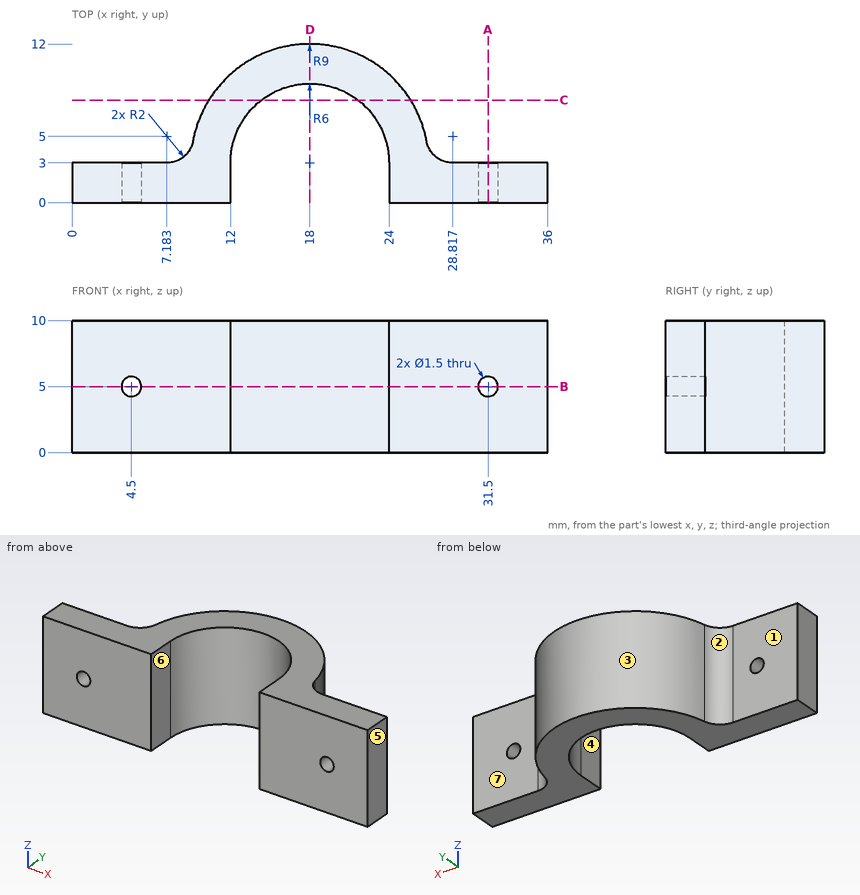
Design review of the part shown in the three views and the two pictorial views. Dimensions are in mm from the part's minimum x, y and z. A direction names the side the tool comes from. Round coordinates to 2 decimals unless told otherwise and drop trailing zeros. Loops run counter-clockwise (first coordinate to the right, second up) from the corner with the lowest first, then second, coordinate; pieces in that order, holes last. Notation, with made-up numbers: (42.25, -18) - (94.25, -18) arc R23 ccw to (94.25, -9) - close; hole circle Ø6 at (-11, 15.5). An arc over 180 degrees is marked (long way). Write each question's results on one line, items separated by ' | '. Start each with the question number.
Q1. Wall thickness on line 1 along Z through (x, y) = (4.5, 2.3); line 2 along X through (y, z) = (1.5, 4); line 3 along X through (y, z) = (1, 5.25): over which ranges is each line inside the solid? List them lowest first. Write a range as [from, to].
Q2. Take a section at D-D on x = 18. Give the boundary of the cut face in (y, z).
Q3. Draft analysis for pull direction X (two halves, no side actions). For the marked faces 1, 2, 3 and 4, state which applies: pulls with the +X half, pulls with the -X half, needs draft (parallel to the pull), parting line crosses it, or undercut.
Q4. Take a section at A-A on x = 31.5. Give the boundary of the cut face in (y, z).
Q5. Insertion check: P1, Ø1.2, axis at x = 31.5, z = 5, coming from the -Y side; P2, Ø3, axis at y = 6.5, z = 8.5, coming from the -X side (1 decimal); P3, Ø4, axis at x = 4, z = 8, coming from the +Y side; P4, Ø3, axis at y = 7.5, z = 6.5, coming from the -X side (1 decimal). Each pin has a flat end and moves straight along its axis. Give the tip position at first contact, or say it passes through.
Q6. Tool access review of the marked faces 5, 6 and 7: name each direction out of +Z, -Z, +X, -X, +Y, -Y from which nothing blocks a thin tool from reaching the whole face with its end or side.
Q7. Take a section at C-C on y = 7.75. Give the boundary of the cut face in (x, z) (1 decimal).
Q8. Take a section at B-B on z = 5. Give the boundary of the cut face in (x, y), plus the area to 3 significant figures.
Data:
1) line 1: z = [0, 4.25], [5.75, 10] | line 2: x = [0, 12], [24, 36] | line 3: x = [0, 3.79], [5.21, 12], [24, 30.79], [32.21, 36]
2) outline: (9, 0) - (12, 0) - (12, 10) - (9, 10) - close
3) face 1: needs draft | face 2: pulls with the -X half | face 3: parting line crosses it | face 4: undercut
4) outline: (0, 0) - (3, 0) - (3, 4.25) - (0, 4.25) - close; (0, 5.75) - (3, 5.75) - (3, 10) - (0, 10) - close
5) P1: passes through | P2: stops at x = 9.2 | P3: stops at y = 3 | P4: stops at x = 9.5
6) face 5: +Z, -Z, +X, +Y, -Y | face 6: +Z, -Z, -Y | face 7: +Z, -Z, +X, +Y
7) outline: (10.4, 0) - (14.3, 0) - (14.3, 10) - (10.4, 10) - close; (21.7, 0) - (25.6, 0) - (25.6, 10) - (21.7, 10) - close
8) outline: (0, 0) - (3.75, 0) - (3.75, 3) - (0, 3) - close; (5.25, 0) - (12, 0) - (12, 3) arc R6 cw to (24, 3) - (24, 0) - (30.75, 0) - (30.75, 3) - (28.82, 3) arc R2 cw to (26.85, 4.64) arc R9 ccw to (9.15, 4.64) arc R2 cw to (7.18, 3) - (5.25, 3) - close; (32.25, 0) - (36, 0) - (36, 3) - (32.25, 3) - close | area: 135 mm²
